```python
from build123d import *

# Parameters (mm, degrees)
F0_R     = 25.4
F1_DEPTH = 12.7
F2_R     = 3.302
F3_DEPTH = 12.7
F4_R     = 3.175
F5_DEPTH = 19.05


# Not quite as in the source:
# - a feature names something its author has since deleted; it is built from what else it names


with BuildPart() as f1:
    # F0 (on Top) → F1 (new body)
    with BuildSketch(Plane.XY):
        Circle(F0_R)
    extrude(amount=F1_DEPTH)

    # F2 (on face) → F3 (cut)
    with BuildSketch(Plane(origin=(0, 0, 0), x_dir=(1, 0, 0), z_dir=(0, 0, -1))):
        Circle(F2_R)
    extrude(amount=-F3_DEPTH, mode=Mode.SUBTRACT)

    # F4 (on face) → F5 (join)
    with BuildSketch(Plane.XY.offset(12.7)):
        with Locations((0, 19.685)):
            Circle(F4_R)
        with Locations((-17.0477100735, 9.8425)):
            Circle(F4_R)
        with Locations((-17.0477100735, -9.8425)):
            Circle(F4_R)
        with Locations((0, -19.685)):
            Circle(F4_R)
        with Locations((17.0477100735, -9.8425)):
            Circle(F4_R)
        with Locations((17.0477100735, 9.8425)):
            Circle(F4_R)
    extrude(amount=F5_DEPTH)


solid = f1.part
```
Could you check a few things on this model? Use its own coordinates, in mm. A direction names the side the tool comes from. Give positions to 0.01 mm unless a question says otherwise; leave off trailing zeros. Write each loop counter-clockwise with the first axis right and the second up, starting at its lowest first coordinate (ties: lowest second). Pieces come first, ordered by that corner, then holes. Notation, with made-up numbers: (-15, 67) -> (-3, 67) arc R27 cw to (-3, 86) -> close; hole circle Ø3 at (38, 89.25). An arc over 180 degrees is marked (long way). Write each question's results on one line, items separated by ' | '.
1. I want a section at C-C, the plane z = 21.5. Count the separate pieces of the cut face and the enclosed holes in it, then the cut area to 3 significant figures.
Check sheet entries:
separate pieces: 6 | enclosed holes: 0 | area: 190 mm²
2. I want a section at A-A, the plane x = 0. Write out the boundary of the cut face in (y, z), then the cut area to 3 significant figures.
Check sheet entries:
outline: (-25.4, 0) -> (-3.3, 0) -> (-3.3, 12.7) -> (-16.51, 12.7) -> (-16.51, 31.75) -> (-22.86, 31.75) -> (-22.86, 12.7) -> (-25.4, 12.7) -> close; (3.3, 0) -> (25.4, 0) -> (25.4, 12.7) -> (22.86, 12.7) -> (22.86, 31.75) -> (16.51, 31.75) -> (16.51, 12.7) -> (3.3, 12.7) -> close | area: 803 mm²
3. I need wall thicknesses on L1, parallel to Y at x = 0, z = 4.25; L2, parallel to Y at x = -17, z = 26.5; L3, parallel to Z at x = 5, y = 18. Which ranges of each line are inside material? Lowest first, please.
Check sheet entries:
L1: y = -25.4 to -3.3, 3.3 to 25.4 | L2: y = -13.02 to -6.67, 6.67 to 13.02 | L3: z = 0 to 12.7
4. I want a section at D-D, the plane z = 10. Write out the boundary of the cut face in (x, y), then the cut area to 3 significant figures.
Check sheet entries:
outline: circle Ø50.8 at (0, 0); hole circle Ø6.6 at (0, 0) | area: 1,990 mm²
5. I want a section at B-B, the plane y = 0. Write out the boundary of the cut face in (x, z), then the cut area to 3 significant figures.
Check sheet entries:
outline: (-25.4, 0) -> (-3.3, 0) -> (-3.3, 12.7) -> (-25.4, 12.7) -> close; (3.3, 0) -> (25.4, 0) -> (25.4, 12.7) -> (3.3, 12.7) -> close | area: 561 mm²
6. Will these pins go through, and if not, where does the flat tip stop? pin 1 Ø3 at (y, z) = (7, 26.5) entering from +X; pin 2 Ø3 at (x, z) = (-2.5, 26.5) entering from -Y; pin 3 Ø12 at (x, z) = (-8.5, 9.5) entering from -Y.
Check sheet entries:
pin 1: stops at x = 19.92 | pin 2: stops at y = -22.7 | pin 3: stops at y = -25.28
7. If we mould it in two halves opening along Y, with no side actions, what happens to faces 1 (the cylindrical face through (-5.506, -24.796, 6.261)), 2 (the flat face through (-17, 10, 31.75)), 3 (the cylindrical face through (-0.688, 16.586, 22.092))? For each: released by +Y, released by -Y, zero draft, split by the parting line, or undercut.
Check sheet entries:
face 1: split by the parting line | face 2: zero draft | face 3: undercut
8. On a 3-axis mill with a long thin cutter (end or side, diameter ignored), from which of +Z, -Z, +X, -X, +Y, -Y can I reach the whole of each face in a straight line? I mean faces 4 (the cylindrical face through (-0.688, -22.784, 22.092)), 5 (the flat face through (0, -20, 31.75)). Say none if no direction works.
Check sheet entries:
face 4: +Z | face 5: +Z, +X, -X, +Y, -Y
